from build123d import *
from OCP.BRepFilletAPI import BRepFilletAPI_MakeChamfer

# Parameters (mm, degrees)
SKETCH1_R           = 4.15
BOSS_EXTRUDE1_DEPTH = 5
SKETCH2_R           = 2.425
BOSS_EXTRUDE2_DEPTH = 80
CUT_EXTRUDE1_DEPTH  = 3
CHAMFER1_SIZE       = 0.5
CHAMFER1_SIZE2      = 0.419549816


with BuildPart() as part:
    # Sketch1 → Boss-Extrude1 (new body)
    with BuildSketch(Plane(origin=(0, 0, 0), x_dir=(1, 0, 0), z_dir=(0, 1, 0))):
        with Locations(Location((0, 0, 0), (0, 0, 270))):
            Circle(SKETCH1_R)
    extrude(amount=BOSS_EXTRUDE1_DEPTH)

    # Sketch2 → Boss-Extrude2 (add)
    with BuildSketch(Plane(origin=(0, 5, 0), x_dir=(1, 0, 0), z_dir=(0, 1, 0))):
        with Locations(Location((0, 0, 0), (0, 0, 270))):
            Circle(SKETCH2_R)
    extrude(amount=BOSS_EXTRUDE2_DEPTH)

    # Sketch3 → Cut-Extrude1 (cut)
    with BuildSketch(Plane.XZ):
        Polygon((0, 2.786041865), (-2.412783031, 1.393020932), (-2.412783031, -1.393020932), (0, -2.786041865), (2.412783031, -1.393020932), (2.412783031, 1.393020932), align=None)
    extrude(amount=-CUT_EXTRUDE1_DEPTH, mode=Mode.SUBTRACT)

    # Chamfer1: one chamfer whose edges measure the first distance from different faces: ONE call of the kernel's chamfer builder (chamfer() names one face for all edges)
    chamfer1_edges_1 = [part.edges().sort_by_distance(p)[0] for p in [
        (0, 0, -4.15),
    ]]
    chamfer1_side_1 = [part.faces().sort_by_distance(p)[0] for p in [
        (0, 0, -4.032620274),
    ]]
    chamfer1_edges_2 = [part.edges().sort_by_distance(p)[0] for p in [
        (0, 5, -4.15),
    ]]
    chamfer1_side_2 = [part.faces().sort_by_distance(p)[0] for p in [
        (0, 2.5, -4.15),
    ]]
    chamfer1_edges_3 = [part.edges().sort_by_distance(p)[0] for p in [
        (0, 85, -2.425),
    ]]
    chamfer1_side_3 = [part.faces().sort_by_distance(p)[0] for p in [
        (0, 45, -2.425),
    ]]
    chamfer1 = BRepFilletAPI_MakeChamfer(part.part.solid().wrapped)
    for e in chamfer1_edges_1:
        chamfer1.Add(CHAMFER1_SIZE, CHAMFER1_SIZE2, e.wrapped, chamfer1_side_1[0].wrapped)  # the first distance lies on this face
    for e in chamfer1_edges_2:
        chamfer1.Add(CHAMFER1_SIZE, CHAMFER1_SIZE2, e.wrapped, chamfer1_side_2[0].wrapped)  # the first distance lies on this face
    for e in chamfer1_edges_3:
        chamfer1.Add(CHAMFER1_SIZE, CHAMFER1_SIZE2, e.wrapped, chamfer1_side_3[0].wrapped)  # the first distance lies on this face
    add(Compound.cast(chamfer1.Shape()), mode=Mode.REPLACE)


solid = part.part
The model under review builds one solid part; all positions refer to its coordinate system, in mm. A direction names the side the tool comes from. Give positions to 0.01 mm unless a question says otherwise; leave off trailing zeros. Write each loop counter-clockwise with the first axis right and the second up, starting at its lowest first coordinate (ties: lowest second). Pieces come first, ordered by that corner, then holes.
1. Tool access review of faces 4 (the cylindrical face through (-2.53, 2.43, -3.29)), 5 (the flat face through (0, 3, 0)), 6 (the flat face through (-2.43, 5, -0.88)): name each direction out of +Z, -Z, +X, -X, +Y, -Y from which nothing blocks a thin tool from reaching the whole face with its end or side.
2. For P1, Ø3, axis at x = 0, y = 56, coming from the +Z side (3 decimals); P2, Ø1, axis at x = -1, y = 71, coming from the -Z side; P3, Ø1.5, axis at x = -3.5, z = 1.5, coming from the +Y side, all flat-tipped, find the tip position at first contact; note any pin that passes through.
3. Draft analysis for pull direction X (two halves, no side actions). For faces 1 (the flat face through (0, 85, 0)), 2 (the cylindrical face through (0.728, 44.194, 2.313)), 3 (the flat face through (-1.19, 1.48, 2.1)), state which applies: +X half, -X half, draft (parallel to the pull), parting line (faces both ways), or undercut.
4. Wall thickness on L1, parallel to Y at x = -0.25, z = 0; L2, parallel to Y at x = -1, z = -3; L3, parallel to X at y = 19, z = -1.5: over which ranges is each line inside the solid? List them lowest first.
5. Add section B-B, the plane y = 67.5. Write out the cut boundary in (x, z) (3 decimals), plus the area to 3 significant figures.
6. Add section A-A, the plane z = 0. Write out the cut boundary in (x, y) (3 decimals).
Worked answers:
1. face 4: +Y, -Y
1. face 5: -Y
1. face 6: +Y
2. P1: stops at z = 2.425
2. P2: stops at z = -2.37
2. P3: stops at y = 5
3. face 1: draft
3. face 2: parting line
3. face 3: undercut
4. L1: y = 3 to 85
4. L2: y = 0 to 5
4. L3: x = -1.91 to 1.91
5. outline: circle Ø4.85 at (0, 0)
5. area: 18.5 mm2
6. outline: (-4.15, 0.42) - (-3.65, 0) - (-2.413, 0) - (-2.413, 3) - (2.413, 3) - (2.413, 0) - (3.65, 0) - (4.15, 0.42) - (4.15, 4.5) - (3.73, 5) - (2.425, 5) - (2.425, 84.5) - (2.005, 85) - (-2.005, 85) - (-2.425, 84.5) - (-2.425, 5) - (-3.73, 5) - (-4.15, 4.5) - close
